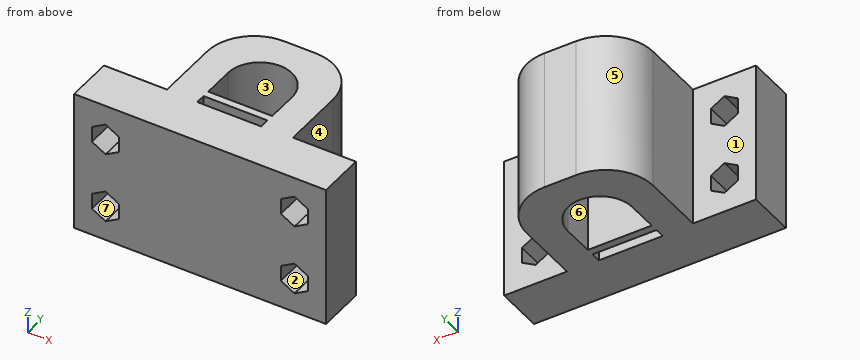
```python
from build123d import *

# Parameters (mm, degrees)
SKETCH1_W           = 50.8
SKETCH1_H           = 28.575
BOSS_EXTRUDE1_DEPTH = 31.75
SKETCH2_W           = 12.7
SKETCH2_H           = 22.225
SKETCH2_W_2         = 12.9
SKETCH2_H_2         = 2
CUT_EXTRUDE1_DEPTH  = 28.575
FILLET2_R           = 9.525
CUT_EXTRUDE2_REACH  = 45.097


with BuildPart() as part:
    # Sketch1 → Boss-Extrude1 (new body)
    with BuildSketch(Plane(origin=(0, 0, 0), x_dir=(1, 0, 0), z_dir=(0, 1, 0))):
        Rectangle(SKETCH1_W, SKETCH1_H)
    extrude(amount=BOSS_EXTRUDE1_DEPTH)

    # Sketch2 → Cut-Extrude1 (cut)
    with BuildSketch(Plane.XY.offset(14.2875)):
        with Locations((-19.05, 20.6375)):
            Rectangle(SKETCH2_W, SKETCH2_H)
        with BuildLine():
            Line((6.45, 12.8), (6.45, 19.05))
            ThreePointArc((6.45, 19.05), (0, 25.5), (-6.45, 19.05))
            Line((-6.45, 19.05), (-6.45, 12.8))
            Line((-6.45, 12.8), (6.45, 12.8))
        make_face()
        with Locations((0, 10.3)):
            Rectangle(SKETCH2_W_2, SKETCH2_H_2)
        with Locations((19.05, 20.6375)):
            Rectangle(SKETCH2_W, SKETCH2_H)
    extrude(amount=-CUT_EXTRUDE1_DEPTH, mode=Mode.SUBTRACT)

    # Fillet2
    fillet2_edges = [part.edges().sort_by_distance(p)[0] for p in [
        (-12.7, 31.75, 0),
        (12.7, 31.75, 0),
    ]]
    fillet(fillet2_edges, radius=FILLET2_R)

    # Sketch9 → Cut-Extrude2 (cut, up to next)
    with BuildSketch(Plane.XZ, mode=Mode.PRIVATE) as cut_extrude2_sk1:
        Polygon((16.3, -5.55603676), (16.3, -8.73146324), (19.05, -10.319176481), (21.8, -8.73146324), (21.8, -5.55603676), (19.05, -3.968323519), align=None)
    cut_extrude2_tool1 = extrude(cut_extrude2_sk1.sketch, amount=-CUT_EXTRUDE2_REACH, mode=Mode.PRIVATE) & part.part
    # Sketch9 → Cut-Extrude2 (cut, up to next)
    with BuildSketch(Plane.XZ, mode=Mode.PRIVATE) as cut_extrude2_sk2:
        Polygon((16.3, 5.55603676), (19.05, 3.968323519), (21.8, 5.55603676), (21.8, 8.73146324), (19.05, 10.319176481), (16.3, 8.73146324), align=None)
    cut_extrude2_tool2 = extrude(cut_extrude2_sk2.sketch, amount=-CUT_EXTRUDE2_REACH, mode=Mode.PRIVATE) & part.part
    # Sketch9 → Cut-Extrude2 (cut, up to next)
    with BuildSketch(Plane.XZ, mode=Mode.PRIVATE) as cut_extrude2_sk3:
        Polygon((-16.3, -8.73146324), (-16.3, -5.55603676), (-19.05, -3.968323519), (-21.8, -5.55603676), (-21.8, -8.73146324), (-19.05, -10.319176481), align=None)
    cut_extrude2_tool3 = extrude(cut_extrude2_sk3.sketch, amount=-CUT_EXTRUDE2_REACH, mode=Mode.PRIVATE) & part.part
    # Sketch9 → Cut-Extrude2 (cut, up to next)
    with BuildSketch(Plane.XZ, mode=Mode.PRIVATE) as cut_extrude2_sk4:
        Polygon((-16.3, 5.55603676), (-16.3, 8.73146324), (-19.05, 10.319176481), (-21.8, 8.73146324), (-21.8, 5.55603676), (-19.05, 3.968323519), align=None)
    cut_extrude2_tool4 = extrude(cut_extrude2_sk4.sketch, amount=-CUT_EXTRUDE2_REACH, mode=Mode.PRIVATE) & part.part
    add(cut_extrude2_tool1.solids().sort_by_distance((19.05, 0, -7.14375))[0], mode=Mode.SUBTRACT)
    add(cut_extrude2_tool2.solids().sort_by_distance((19.05, 0, 7.14375))[0], mode=Mode.SUBTRACT)
    add(cut_extrude2_tool3.solids().sort_by_distance((-19.05, 0, -7.14375))[0], mode=Mode.SUBTRACT)
    add(cut_extrude2_tool4.solids().sort_by_distance((-19.05, 0, 7.14375))[0], mode=Mode.SUBTRACT)


solid = part.part
```
Can you work these out from the model? Positions are in its coordinate system, mm. Face numbers are marked on the shaded views. A direction names the side the tool comes from. Give positions to 0.01 mm unless a question says otherwise; leave off trailing zeros. Loops run counter-clockwise (first coordinate to the right, second up) from the corner with the lowest first, then second, coordinate; pieces in that order, holes last. Notation, with made-up numbers: M -31,-38.5 L -15,-38.5 A30 cw -15,-4.5 Z; hole C -8,59 d5. An arc over 180 degrees is marked long. Use CSV: the item, a comma, the result in double quotes. Start each with the question number.
1. If I drill on L1, parallel to Y at x = -1.5, z = 2.25; L2, parallel to Y at x = -0.5, z = 11.75; L3, parallel to X at y = 14, z = 0.25, over which ranges is the centre line in solid material (lowest first)?
2. Imagine slicing it at C-C, the plane z = -1. Write out the boundary of the cut face in (x, y) (3 decimals).
3. On a 3-axis mill with a long thin cutter (end or side, diameter ignored), from which of +Z, -Z, +X, -X, +Y, -Y can I reach the whole of each face in a straight line? I mean the marked faces 1, 2, 3 and 4. Say none if no direction works.
4. For P1, Ø4, axis at x = 17.5, z = 3, coming from the +Y side (3 decimals); P2, Ø3, axis at y = 22.5, z = -3, coming from the +X side; P3, Ø1, axis at y = 25, z = -7, coming from the -X side, each with a flat end and sliding along its axis, tell me the tip position at first contact or that it passes through.
5. Imagine slicing it at B-B, the plane y = 16.5. Write out the boundary of the cut face in (x, z).
6. Imagine slicing it at A-A, the plane x = 0. Write out the boundary of the cut face in (y, z), plus the area to 3 significant figures.
7. If we mould it in two halves opening along Y, with no side actions, what happens to the marked faces 5, 6 and 7? For each: released by +Y, released by -Y, zero draft, split by the parting line, or undercut.
8. Imagine slicing it at D-D, the plane y = 8.5. Write out the boundary of the cut face in (x, z).
Response values:
1,L1,"0 to 9.3, 11.3 to 12.8, 25.32 to 31.75"
1,L2,"0 to 9.3, 11.3 to 12.8, 25.48 to 31.75"
1,L3,"-12.7 to -6.45, 6.45 to 12.7"
2,outline,"M -25.4,0 L 25.4,0 L 25.4,9.525 L 12.7,9.525 L 12.7,22.225 A9.525 ccw 3.175,31.75 L -3.175,31.75 A9.525 ccw -12.7,22.225 L -12.7,9.525 L -25.4,9.525 Z; hole M -6.45,9.3 L 6.45,9.3 L 6.45,11.3 L -6.45,11.3 Z; hole M -6.45,12.8 L 6.45,12.8 L 6.45,19.05 A6.45 ccw -6.45,19.05 Z"
3,face 1,"+Z, -Z, -X, +Y"
3,face 2,"+Y, -Y"
3,face 3,"+Z, -Z"
3,face 4,"+Z, -Z, +X, +Y"
4,P1,"y = 9.525"
4,P2,"x = 12.7"
4,P3,"x = -12.42"
5,outline,"M -12.7,-14.29 L -6.45,-14.29 L -6.45,14.29 L -12.7,14.29 Z; M 6.45,-14.29 L 12.7,-14.29 L 12.7,14.29 L 6.45,14.29 Z"
6,outline,"M 0,-14.29 L 9.3,-14.29 L 9.3,14.29 L 0,14.29 Z; M 11.3,-14.29 L 12.8,-14.29 L 12.8,14.29 L 11.3,14.29 Z; M 25.5,-14.29 L 31.75,-14.29 L 31.75,14.29 L 25.5,14.29 Z"
6,area,"487 mm^2"
7,face 5,"released by +Y"
7,face 6,"undercut"
7,face 7,"zero draft"
8,outline,"M -25.4,-14.29 L 25.4,-14.29 L 25.4,14.29 L -25.4,14.29 Z; hole M -21.8,-8.73 L -19.05,-10.32 L -16.3,-8.73 L -16.3,-5.56 L -19.05,-3.97 L -21.8,-5.56 Z; hole M -21.8,5.56 L -19.05,3.97 L -16.3,5.56 L -16.3,8.73 L -19.05,10.32 L -21.8,8.73 Z; hole M 16.3,-8.73 L 19.05,-10.32 L 21.8,-8.73 L 21.8,-5.56 L 19.05,-3.97 L 16.3,-5.56 Z; hole M 16.3,5.56 L 19.05,3.97 L 21.8,5.56 L 21.8,8.73 L 19.05,10.32 L 16.3,8.73 Z"
